Verification items for the finished model (mm, model axes). A direction names the side the tool comes from. Round coordinates to 2 decimals unless told otherwise and drop trailing zeros. Loops run counter-clockwise (first coordinate to the right, second up) from the corner with the lowest first, then second, coordinate; pieces in that order, holes last. Notation, with made-up numbers: M -16,46 L 22,46 A21 cw 22,82 Z; hole C 40.5,-13 d2. An arc over 180 degrees is marked long. Write item = value, one per line. Start each with the question number.
from build123d import *
from build123d.topology import SkipClean

# Parameters (mm, degrees)
SKETCH_1_R          = 40
SKETCH_1_R_2        = 31.75
EXTRUDE_1_DEPTH     = 4
EXTRUDE_START       = -4
SKETCH_2_R          = 1.75
EXTRUDE_2_DEPTH     = 4
CUT_EXTRUDE_2_DEPTH = 57.709787515
SKETCH_4_R          = 1.75
EXTRUDE_3_DEPTH     = 4
SKETCH_5_R          = 34.75
SKETCH_5_R_2        = 31.75
EXTRUDE_4_DEPTH     = 4
CUT_EXTRUDE_3_DEPTH = 59.310727346
EXTRUDE_5_DEPTH     = 4
EXTRUDE_6_DEPTH     = 1
CUT_EXTRUDE_START   = -2
CUT_EXTRUDE_4_DEPTH = 2
CUT_EXTRUDE_START_2 = -1
CUT_EXTRUDE_5_DEPTH = 1
CHAMFER_1_SIZE      = 1
SKETCH_11_W         = 4.981706152
SKETCH_11_H         = 1.5
CUT_EXTRUDE_6_DEPTH = 4
CHAMFER_2_SIZE      = 0.5
SKETCH_12_W         = 4
SKETCH_12_H         = 3.514481439
CUT_EXTRUDE_7_DEPTH = 4
CHAMFER_3_SIZE      = 0.5
SKETCH_13_W         = 1
SKETCH_13_H         = 1
CUT_EXTRUDE_8_DEPTH = 1


with BuildPart() as part:
    # 草图1 → 凸台-拉伸1 (new body)
    with BuildSketch(Plane.XY):
        Circle(SKETCH_1_R)
        Circle(SKETCH_1_R_2, mode=Mode.SUBTRACT)
    extrude(amount=EXTRUDE_1_DEPTH)

    # 草图2 → 凸台-拉伸2 (add)
    # profile 1 of 2: a face of its own
    with BuildSketch(Plane.XY.offset(4).offset(EXTRUDE_START)):
        with BuildLine():
            Line((-36.962769782, -22.533389671), (-34.351514644, -20.493253565))
            ThreePointArc((-34.351514644, -20.493253565), (-31.520430144, -24.626459013), (-28.194899891, -28.373361101))
            Line((-28.194899891, -28.373361101), (-30.806155028, -30.413497207))
            ThreePointArc((-30.806155028, -30.413497207), (-37.824516173, -29.551750816), (-36.962769782, -22.533389671))
        make_face()
        with Locations((-33.884462405, -26.473443439)):
            Circle(SKETCH_2_R, mode=Mode.SUBTRACT)
    # profile 2 of 2: a face of its own
    with BuildSketch(Plane.XY.offset(4).offset(EXTRUDE_START)):
        with BuildLine():
            Line((30.806155028, -30.413497207), (28.194899891, -28.373361101))
            ThreePointArc((28.194899891, -28.373361101), (31.520430144, -24.626459013), (34.351514644, -20.493253565))
            Line((34.351514644, -20.493253565), (36.962769782, -22.533389671))
            ThreePointArc((36.962769782, -22.533389671), (37.824516173, -29.551750816), (30.806155028, -30.413497207))
        make_face()
        with Locations((33.884462405, -26.473443439)):
            Circle(SKETCH_2_R, mode=Mode.SUBTRACT)
    extrude(amount=EXTRUDE_2_DEPTH)

    # 草图3 → 切除-拉伸2 (cut, through all)
    with BuildSketch(Plane.XY.offset(4)):
        with BuildLine():
            Line((-24, -32), (-15.370426149, -32))
            ThreePointArc((-15.370426149, -32), (0, -35.5), (15.370426149, -32))
            Line((15.370426149, -32), (24, -32))
            ThreePointArc((24, -32), (0, -40), (-24, -32))
        make_face()
    extrude(amount=-CUT_EXTRUDE_2_DEPTH, mode=Mode.SUBTRACT)

    # 草图4 → 凸台-拉伸3 (add)
    # profile 1 of 2: a face of its own
    with BuildSketch(Plane.XY.offset(4).offset(EXTRUDE_START)):
        with BuildLine():
            Line((-37.239092363, 26.5), (-29.962476533, 26.5))
            ThreePointArc((-29.962476533, 26.5), (-33.86444566, 21.288478578), (-36.869317712, 15.513007814))
            Line((-36.869317712, 15.513007814), (-39.739092363, 17.169872981))
            ThreePointArc((-39.739092363, 17.169872981), (-42.068721494, 22.794095226), (-37.239092363, 26.5))
        make_face()
        with Locations((-37.239092363, 21.5)):
            Circle(SKETCH_4_R, mode=Mode.SUBTRACT)
    # profile 2 of 2: a face of its own
    with BuildSketch(Plane.XY.offset(4).offset(EXTRUDE_START)):
        with BuildLine():
            Line((39.739092363, 17.169872981), (36.869317712, 15.513007814))
            ThreePointArc((36.869317712, 15.513007814), (33.86444566, 21.288478578), (29.962476533, 26.5))
            Line((29.962476533, 26.5), (37.239092363, 26.5))
            ThreePointArc((37.239092363, 26.5), (42.068721494, 22.794095226), (39.739092363, 17.169872981))
        make_face()
        with Locations((37.239092363, 21.5)):
            Circle(SKETCH_4_R, mode=Mode.SUBTRACT)
    extrude(amount=EXTRUDE_3_DEPTH)

    # 草图5 → 凸台-拉伸4 (add)
    with BuildSketch(Plane(origin=(0, 0, 4), x_dir=(-1, 0, 0), z_dir=(0, 0, -1))):
        Circle(SKETCH_5_R)
        Circle(SKETCH_5_R_2, mode=Mode.SUBTRACT)
    extrude(amount=-EXTRUDE_4_DEPTH)

    # 草图6 → 切除-拉伸3 (cut, through all)
    with SkipClean():  # the faces are left unmerged after this step: merging them gives an invalid solid
        with BuildSketch(Plane.XY.offset(4)):
            with BuildLine():
                Line((-15.045698836, -31.323943662), (-13.746789584, -28.61971831))
                ThreePointArc((-13.746789584, -28.61971831), (-5.692283606, -31.235563183), (2.767194832, -31.629181664))
                Line((2.767194832, -31.629181664), (3.02866206, -34.617765759))
                ThreePointArc((3.02866206, -34.617765759), (-6.230137175, -34.18695498), (-15.045698836, -31.323943662))
            make_face()
        extrude(amount=CUT_EXTRUDE_3_DEPTH, mode=Mode.SUBTRACT)

    # 草图7 → 凸台-拉伸5 (add)
    with SkipClean():  # the faces are left unmerged after this step: merging them gives an invalid solid
        with BuildSketch(Plane.XY.offset(4)):
            with BuildLine():
                Line((-2, 39.949968711), (-2, 34.692398303))
                ThreePointArc((-2, 34.692398303), (0, 34.75), (2, 34.692398303))
                Line((2, 34.692398303), (2, 39.949968711))
                ThreePointArc((2, 39.949968711), (0, 40), (-2, 39.949968711))
            make_face()
        extrude(amount=EXTRUDE_5_DEPTH)

    # 草图8 → 凸台-拉伸6 (add)
    with SkipClean():  # the faces are left unmerged after this step: merging them gives an invalid solid
        with BuildSketch(Plane.XY.offset(8)):
            with BuildLine():
                Line((-0.5, 39.996874878), (-0.5, 31.746062748))
                ThreePointArc((-0.5, 31.746062748), (0, 31.75), (0.5, 31.746062748))
                Line((0.5, 31.746062748), (0.5, 39.996874878))
                ThreePointArc((0.5, 39.996874878), (0, 40), (-0.5, 39.996874878))
            make_face()
        extrude(amount=EXTRUDE_6_DEPTH)

    # 草图9 → 切除-拉伸4 (cut)
    with SkipClean():  # the faces are left unmerged after this step: merging them gives an invalid solid
        with BuildSketch(Plane.XY.offset(4).offset(CUT_EXTRUDE_START)):
            with BuildLine():
                Line((-15.045698836, -31.323943662), (-15.370426149, -32))
                ThreePointArc((-15.370426149, -32), (-6.364600567, -34.924802929), (3.094028868, -35.364911782))
                Line((3.094028868, -35.364911782), (3.02866206, -34.617765759))
                ThreePointArc((3.02866206, -34.617765759), (-6.230137175, -34.18695498), (-15.045698836, -31.323943662))
            make_face()
        extrude(amount=CUT_EXTRUDE_4_DEPTH, mode=Mode.SUBTRACT)

    # 草图10 → 切除-拉伸5 (cut)
    with BuildSketch(Plane.XY.offset(4).offset(CUT_EXTRUDE_START_2)):
        with BuildLine():
            Line((3.02866206, -34.617765759), (2.767194832, -31.629181664))
            ThreePointArc((2.767194832, -31.629181664), (-5.692283606, -31.235563183), (-13.746789584, -28.61971831))
            Line((-13.746789584, -28.61971831), (-15.045698836, -31.323943662))
            ThreePointArc((-15.045698836, -31.323943662), (-6.230137175, -34.18695498), (3.02866206, -34.617765759))
        make_face()
    extrude(amount=CUT_EXTRUDE_5_DEPTH, mode=Mode.SUBTRACT)

    # 倒角1
    # the kernel refuses this chamfer: 1 mm, written as the material it adds along each edge
    with BuildSketch(Plane(origin=(0, 0, 2), x_dir=(0.1605769660987581, -0.9870233218918986, 0), z_dir=(0.9870233218918986, 0.1605769660987581, 0))) as chamfer_1_piece_1_section:
        Polygon((34.75 + CHAMFER_1_SIZE, 0), (34.75, -CHAMFER_1_SIZE), (34.75, 0), align=None)
    chamfer_1_piece_1 = revolve(axis=Axis((0, 0, 2), (0, 0, -1)), revolution_arc=39.1369501, mode=Mode.PRIVATE)
    chamfer_1_piece_1 = chamfer_1_piece_1 & Plane(origin=(0, 0, 2), x_dir=(-0.4329697506743493, -0.9014084507042253, 0), z_dir=(0, 0, 1)) * Cylinder(35.5, 143, mode=Mode.PRIVATE)
    add(chamfer_1_piece_1)

    # 草图11 → 切除-拉伸6 (cut)
    with BuildSketch(Plane.XY.offset(8)):
        with Locations((9.990853076, -33.180996154)):
            Rectangle(SKETCH_11_W, SKETCH_11_H)
    extrude(amount=-CUT_EXTRUDE_6_DEPTH, mode=Mode.SUBTRACT)

    # 倒角2
    chamfer_2_edges = [part.edges().sort_by_distance(p)[0] for p in [
        (7.5, -32.430996154, 6),
    ]]
    chamfer(chamfer_2_edges, length=CHAMFER_2_SIZE)

    # 草图12 → 切除-拉伸7 (cut)
    with BuildSketch(Plane.XY.offset(4)):
        with Locations((4, 32.935157584)):
            Rectangle(SKETCH_12_W, SKETCH_12_H)
    extrude(amount=CUT_EXTRUDE_7_DEPTH, mode=Mode.SUBTRACT)

    # 倒角3
    # the kernel refuses this chamfer: 0.630512845, 0.5, 0.471250803, 0.431912073 mm, written as the material it takes off along each edge
    with BuildSketch(Plane(origin=(2, 31.686945261, 9.285841494), x_dir=(0, 1, 0), z_dir=(0, 0, -1))) as chamfer_3_piece_1:
        with BuildLine():
            Line((CHAMFER_3_SIZE, 0), (0.026344876, -0.473655124))
            ThreePointArc((0.026344876, -0.473655124), (0.014426752, -0.243437323), (0, 0))
            Line((0, 0), (CHAMFER_3_SIZE, 0))
        make_face()
    extrude(amount=5.285841494, mode=Mode.SUBTRACT)
    with BuildSketch(Plane(origin=(6, 34.228095185, 9.285841494), x_dir=(0.9838938998328699, -0.17875344436308485, 0), z_dir=(0, 0, -1))) as chamfer_3_piece_2:
        with BuildLine():
            Line((0.430053019, 0), (CHAMFER_3_SIZE * 0.178753444363, CHAMFER_3_SIZE * 0.983893899833))
            Line((CHAMFER_3_SIZE * 0.178753444363, CHAMFER_3_SIZE * 0.983893899833), (0, 0))
            ThreePointArc((0, 0), (0.220718474, -0.000664812), (0.430053019, 0))
        make_face()
    extrude(amount=5.285841494, mode=Mode.SUBTRACT)
    with BuildSketch(Plane(origin=(6, 31.177916864, 4), x_dir=(0, 1, 0), z_dir=(0, 0, 1))) as chamfer_3_piece_3:
        with BuildLine():
            Line((CHAMFER_3_SIZE, 0), (-0.127287982, -0.627287982))
            ThreePointArc((-0.127287982, -0.627287982), (-0.064155933, -0.324269183), (0, 0))
            Line((0, 0), (CHAMFER_3_SIZE, 0))
        make_face()
    extrude(amount=5.653107156, mode=Mode.SUBTRACT)

    # 草图13 → 切除-拉伸8 (cut)
    with BuildSketch(Plane.XY.offset(8)):
        with Locations((0, 32.246062748)):
            Rectangle(SKETCH_13_W, SKETCH_13_H)
    extrude(amount=CUT_EXTRUDE_8_DEPTH, mode=Mode.SUBTRACT)


solid = part.part
1. Section check B-B, the plane x = 4.5. Enter the section's corners in (y, z).
2. Tool access check on faces 5 (the flat face through (-14.367, -29.911, 5.085)), 6 (the cylindrical face through (26.131, -30.285, 1.972)), 7 (the flat face through (35.64, -21.5, 1.97)), 8 (the flat face through (10, -32.431, 6)). Record the directions out of +Z, -Z, +X, -X, +Y, -Y that give a thin tool (end or side, any length) a straight path to the whole face; none if there is none.
3. Gauge pin test, flat ends, axial feed: P1, Ø1.2, axis at x = 1.5, y = 36.5, coming from the +Z side; P2, Ø2, axis at y = 37, z = 7, coming from the +X side; P3, Ø4, axis at x = 37.24, y = 21.5, coming from the +Z side; P4, Ø2, axis at x = -37.24, y = 21.5, coming from the -Z side. Record the tip position at first contact, or that the pin passes through.
4. Section check A-A, the plane z = 5. Enter the section's corners in (x, y), and give its area (3 significant figures).
5. Mould release check, pull along Y, two halves, no side actions. Record for faces 1 (the cylindrical face through (-32.94, -25, 1.97)), 2 (the flat face through (32, 0, 8)), 3 (the cylindrical face through (34.544, 3.775, 5.972)), 4 (the flat face through (-38.284, 16.33, 1.972)): pulls with the +Y half, pulls with the -Y half, needs draft (parallel to the pull), parting line crosses it, or undercut.
6. Section check C-C, the plane y = -19.5. Enter the section's corners in (x, z), and give its area (3 significant figures).
7. Thickness scan on line 1 (X direction, y = 0, z = 1.2); line 2 (Y direction, x = -36.5, z = 2.75); line 3 (X direction, y = 37.5, z = 7.25). Record the ranges inside material, lowest first.
8. Section check D-D, the plane y = 21.5. Enter the section's corners in (x, z), and give its area (3 significant figures).
Computed values:
q1.outline = M -35.21,0 L -31.43,0 L -31.43,8 L -34.46,8 L -34.46,4 L -35.21,4 Z; M 31.43,0 L 39.75,0 L 39.75,4 L 31.43,4 Z
q2.face_5 = +Z, -Y
q2.face_6 = +Z, -Z, -Y
q2.face_7 = +Z, -Z, +X
q2.face_8 = +Z, +X, -Y
q3.P1 = 8
q3.P2 = 2
q3.P3 = 4
q3.P4 = through
q4.outline = M -15.05,-31.32 L -13.75,-28.62 A31.75 cw 1.53,31.71 L 2,32.19 L 2,39.95 A40 ccw -2,39.95 L -2,34.69 A34.75 ccw Z; M 2.77,-31.63 L 3.03,-34.62 A34.75 ccw 7.5,-33.93 L 7.5,-32.93 L 8,-32.43 L 12.48,-32.43 A34.75 ccw 6.42,34.15 L 6,33.73 L 6,31.68 L 6.63,31.05 A31.75 cw Z
q4.area = 578 mm2
q5.face_1 = undercut
q5.face_2 = needs draft
q5.face_3 = parting line crosses it
q5.face_4 = undercut
q6.outline = M -34.92,0 L -25.06,0 L -25.06,8 L -28.76,8 L -28.76,4 L -34.92,4 Z; M 25.06,0 L 34.92,0 L 34.92,4 L 28.76,4 L 28.76,8 L 25.06,8 Z
q6.area = 109 mm2
q7.line_1 = -40 to -31.75, 31.75 to 40
q7.line_2 = -30.73 to -22.17, -16.36 to 19.91, 23.09 to 26.5
q7.line_3 = -2 to 2
q8.outline = M -42.24,0 L -38.99,0 L -38.99,4 L -42.24,4 Z; M -35.49,0 L -23.36,0 L -23.36,8 L -27.3,8 L -27.3,4 L -35.49,4 Z; M 23.36,0 L 35.49,0 L 35.49,4 L 27.3,4 L 27.3,8 L 23.36,8 Z; M 38.99,0 L 42.24,0 L 42.24,4 L 38.99,4 Z
q8.area = 155 mm2
